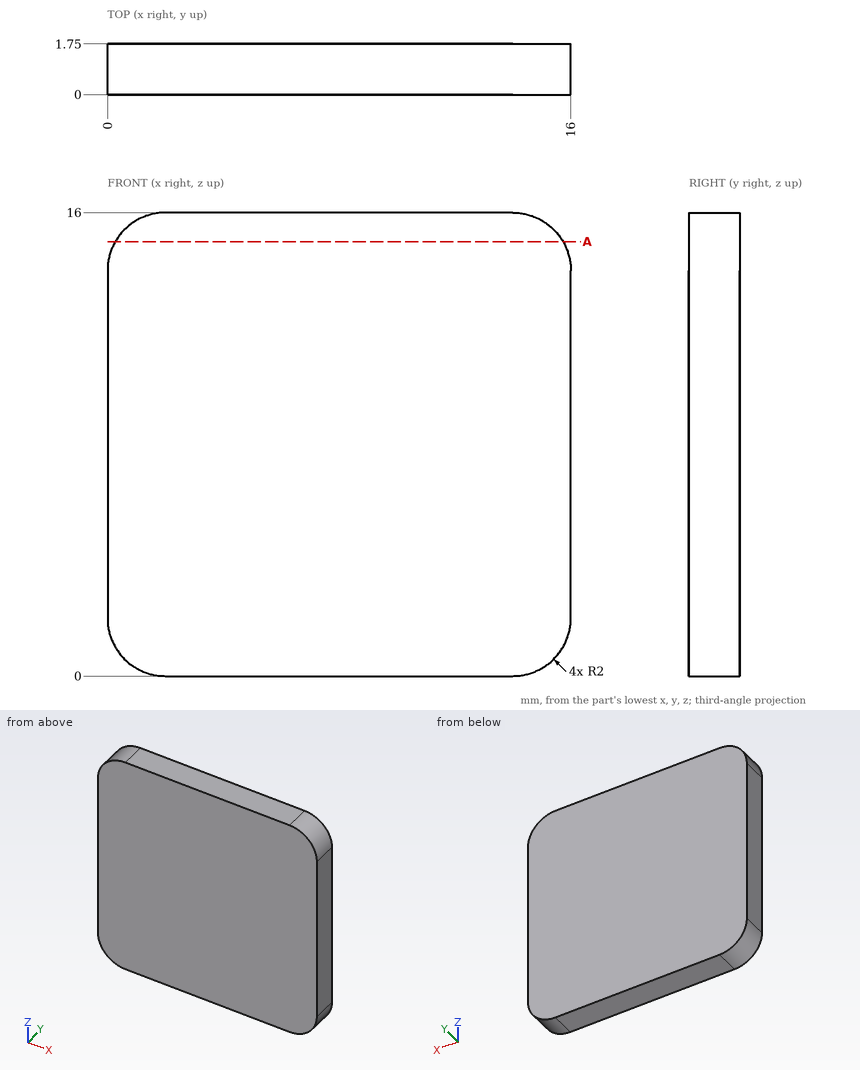
Source: three-view drawing plus pictorial views. Frame: mm from the lowest corner of the part. Round coordinates to 2 decimals unless told otherwise and drop trailing zeros. Loops run counter-clockwise (first coordinate to the right, second up) from the corner with the lowest first, then second, coordinate; pieces in that order, holes last.
Q1. Section A-A on z = 15. Return loops of the section in (x, y).
Q2. Pin query (flat end, axial travel): P1, Ø8, axis at x = 9, z = 4, coming from the -Y side. Return the tip coordinate at first contact, or that it passes through.
Q3. Material intervals for L1, parallel to Z at x = 14.5, y = 0.35; L2, parallel to Z at x = 1.75, y = 1.15, sorted ascending.
Evaluation:
1. outline: (0.27, 0) - (15.73, 0) - (15.73, 1.75) - (0.27, 1.75) - close
2. P1: stops at y = 0
3. L1: z = 0.06 to 15.94
3. L2: z = 0.02 to 15.98
